from build123d import *

# Parameters (mm, degrees)
SKETCH2_R           = 1.8
BOSS_EXTRUDE1_DEPTH = 20


with BuildPart() as part:
    # Sketch2 → Boss-Extrude1 (new body)
    with BuildSketch(Plane.XY):
        with BuildLine():
            ThreePointArc((-60.998373194, 25.417629235), (-69.501790799, 24.76016427), (-65.048841754, 17.486127155))
            Line((-65.048841754, 17.486127155), (-65.05, -37.513872835))
            ThreePointArc((-65.05, -37.513872835), (-69.522135955, -44.749940812), (-61.05, -45.513872835))
            ThreePointArc((-61.05, -45.513872835), (-55.750093871, -47.341941191), (-52.084473347, -43.1))
            Line((-52.084473347, -43.1), (-36.9, -43.1))
            Line((-36.9, -43.1), (36.9, -43.1))
            Line((36.9, -43.1), (52.070291173, -43.1))
            ThreePointArc((52.070291173, -43.1), (55.684136776, -47.459825117), (61.05, -45.65))
            ThreePointArc((61.05, -45.65), (69.522135955, -44.886067977), (65.05, -37.65))
            Line((65.05, -37.65), (65.05, 17.35))
            ThreePointArc((65.05, 17.35), (69.522135955, 24.586067977), (61.05, 25.35))
            ThreePointArc((61.05, 25.35), (57.099855684, 27.349751435), (53.110619235, 25.429168588))
            Line((53.110619235, 25.429168588), (40.839380765, 35.020831412))
            ThreePointArc((40.839380765, 35.020831412), (38.528357482, 42.827414929), (31.9, 38.1))
            Line((31.9, 38.1), (-31.9, 38.1))
            ThreePointArc((-31.9, 38.1), (-38.528357482, 42.827414929), (-40.839380765, 35.020831412))
            Line((-40.839380765, 35.020831412), (-53.110619235, 25.429168588))
            ThreePointArc((-53.110619235, 25.429168588), (-57.057314719, 27.349994649), (-60.998373194, 25.417629235))
        make_face()
        with Locations((-65.05, -42.513872835)):
            Circle(SKETCH2_R, mode=Mode.SUBTRACT)
        with Locations((-57.05, -42.513872835)):
            Circle(SKETCH2_R, mode=Mode.SUBTRACT)
        with Locations((-36.9, -38.1)):
            Circle(SKETCH2_R, mode=Mode.SUBTRACT)
        with Locations((36.9, -38.1)):
            Circle(SKETCH2_R, mode=Mode.SUBTRACT)
        with Locations((57.05, -42.65)):
            Circle(SKETCH2_R, mode=Mode.SUBTRACT)
        with Locations((65.05, -42.65)):
            Circle(SKETCH2_R, mode=Mode.SUBTRACT)
        with Locations((-65.048841754, 22.486127155)):
            Circle(SKETCH2_R, mode=Mode.SUBTRACT)
        with Locations((-57.05, 22.35)):
            Circle(SKETCH2_R, mode=Mode.SUBTRACT)
        with Locations((-36.9, 38.1)):
            Circle(SKETCH2_R, mode=Mode.SUBTRACT)
        with Locations((57.05, 22.35)):
            Circle(SKETCH2_R, mode=Mode.SUBTRACT)
        with Locations((65.05, 22.35)):
            Circle(SKETCH2_R, mode=Mode.SUBTRACT)
        with Locations((36.9, 38.1)):
            Circle(SKETCH2_R, mode=Mode.SUBTRACT)
    extrude(amount=BOSS_EXTRUDE1_DEPTH)


solid = part.part
Check sheet for the modelled part. Datum: model origin and axes. Units: mm. Round coordinates to 2 decimals unless told otherwise and drop trailing zeros. Write each loop counter-clockwise with the first axis right and the second up, starting at its lowest first coordinate (ties: lowest second). Pieces come first, ordered by that corner, then holes. Notation, with made-up numbers: (50, -25.5) - (76, -25.5) arc R11 ccw to (76, -20.5) - close; hole circle Ø3 at (75, 73.5). An arc over 180 degrees is marked (long way). Return JSON: item names as keys, results as strings.
Q1. Cross-section at A-A (x = 36.9). Record the boundary of the cut face in (y, z), then the cut area to 3 significant figures.
Returned:
{"outline": "(-43.1, 0) - (-39.9, 0) - (-39.9, 20) - (-43.1, 20) - close; (-36.3, 0) - (36.3, 0) - (36.3, 20) - (-36.3, 20) - close; (39.9, 0) - (43.1, 0) - (43.1, 20) - (39.9, 20) - close", "area": "1,580 mm²"}
Q2. Cross-section at C-C (z = 18.5). Give the number of separate pieces and of enclosed holes in the cut face, then the cut area to 3 significant figures.
Returned:
{"separate pieces": "1", "enclosed holes": "12", "area": "10,300 mm²"}
Q3. Draft check along Y on faces 1 (the cylindrical face through (-66.48, -43.61, 9.86)), 2 (the flat face through (0, 38.1, 10)). Enter one of: released by +Y, released by -Y, zero draft, split by the parting line, or undercut.
Returned:
{"face 1": "undercut", "face 2": "released by +Y"}
Q4. Cross-section at D-D (y = 1.5). Record the boundary of the cut face in (x, z), then the cut area to 3 significant figures.
Returned:
{"outline": "(-65.05, 0) - (65.05, 0) - (65.05, 20) - (-65.05, 20) - close", "area": "2,600 mm²"}
Q5. Depth check by flat-ended pin: P1, Ø1.5, axis at x = -55, z = 12.5, coming from the +Y side; P2, Ø6, axis at x = 14, z = 6, coming from the +Y side; P3, Ø2, axis at x = -45, z = 5.5, coming from the +Y side; P4, Ø2, axis at x = 36.9, y = -38.1, coming from the -Z side. Enter the tip coordinate at first touch or a pass-through.
Returned:
{"P1": "stops at y = 27.18", "P2": "stops at y = 38.1", "P3": "stops at y = 32.55", "P4": "passes through"}
Q6. Scan lines: L1, parallel to Y at x = -57.05, z = 4.75; L2, parallel to Y at x = 36.9, z = 9.5; L3, parallel to X at y = -38.5, z = 3.75 (3 decimals). Record each from-to range of solid material in increasing order. Write a range as from..to.
Returned:
{"L1": "y = -47.51..-44.31, -40.71..20.55, 24.15..27.35", "L2": "y = -43.1..-39.9, -36.3..36.3, 39.9..43.1", "L3": "x = -68.031..-38.655, -35.145..35.145, 38.655..67.839"}
Q7. Cross-section at B-B (x = -57.05). Record the boundary of the cut face in (y, z), then the cut area to 3 significant figures.
Returned:
{"outline": "(-47.51, 0) - (-44.31, 0) - (-44.31, 20) - (-47.51, 20) - close; (-40.71, 0) - (20.55, 0) - (20.55, 20) - (-40.71, 20) - close; (24.15, 0) - (27.35, 0) - (27.35, 20) - (24.15, 20) - close", "area": "1,350 mm²"}
